Autodesk Inventor part; units mm, degrees
ref_plane "YZ Plane" through (0, 0, 0) normal (1, 0, 0) x (0, 1, 0)
ref_plane "XZ Plane" through (0, 0, 0) normal (0, 1, 0) x (-1, 0, 0)
ref_plane "XY Plane" through (0, 0, 0) normal (0, 0, 1) x (1, 0, 0)
sketch "Sketch1" plane through (0, 0, 0) normal (1, 0, 0) x (0, 1, 0)
  circle A0 centre (0, 0) radius 12.5
  circle A1 centre (-15.5, -15.5) radius 1.75
  circle A2 centre (15.5, -15.5) radius 1.75
  circle A3 centre (15.5, 15.5) radius 1.75
  circle A4 centre (-15.5, 15.5) radius 1.75
  line L0 (21.5, -21.5) -> (-21.5, -21.5)
  line L1 (-21.5, -21.5) -> (-21.5, 21.5)
  line L2 (-21.5, 21.5) -> (21.5, 21.5)
  line L3 (21.5, 21.5) -> (21.5, -21.5)
  line L4 (21.5, -21.5) -> (-21.5, 21.5) construction
  line L5 (-21.5, -21.5) -> (21.5, 21.5) construction
  dimension "d2" = 360
  dimension "d4" = 3.5
  dimension "d5" = 25
  dimension "d6" = 31
  dimension "d7" = 43
extrude "Extrusion1" add sketch "Sketch1" along normal blind 4
sketch "Sketch5" plane through (0, 21.5, 21.5) normal (0, 1, 0) x (1, 0, 0)
  line L0 (0, 43) -> (0, 0)
  line L1 (0, 0) -> (4, 0)
  line L2 (4, 43) -> (4, 0)
  line L3 (0, 43) -> (4, 43)
  line L4 (0, 43) -> (4, 43)
  line L5 (0, 43) -> (-18, 43)
  line L6 (-18, 43) -> (-18, 58)
  line L7 (-18, 58) -> (-15, 58)
  line L8 (-15, 58) -> (-15, 48)
  line L9 (-15, 48) -> (4, 48)
  line L10 (4, 48) -> (4, 43)
  line L11 (0, 0) -> (-18, 0)
  line L12 (-18, 0) -> (-18, -15)
  line L13 (-18, -15) -> (-15, -15)
  line L14 (-15, -15) -> (-15, -5)
  line L15 (-15, -5) -> (4, -5)
  line L16 (4, -5) -> (4, 0)
  line L17 (4, 43) -> (4, 0)
  point P0 (0, 21.5)
  dimension "d17" = 5
  dimension "d18" = 3
  dimension "d19" = 10
  dimension "d23" = 22
extrude "Extrusion4" add sketch "Sketch5" against normal up to surface (43 mm away) contours L5 L6 L7 L8 L9 L10 L3 | L1 L16 L15 L14 L13 L12 L11
sketch "Sketch6" plane through (-15, 21.5, 36.5) normal (1, 0, 0) x (0, 0, -1)
  line L0 (0, -43) -> (10, -43)
  line L1 (10, 0) -> (10, -43)
  line L2 (0, 0) -> (10, 0)
  line L3 (0, 0) -> (0, -43)
  line L4 (63, -43) -> (73, -43)
  line L5 (73, 0) -> (73, -43)
  line L6 (63, 0) -> (73, 0)
  line L7 (63, 0) -> (63, -43)
  point P0 (36.5, -21.5)
  point P1 (5, -6.5)
  point P2 (5, -36.5)
  point P3 (68, -36.5)
  point P4 (68, -6.5)
  point P5 (5, 0)
  point P6 (5, -43)
  point P7 (68, -43)
  point P8 (68, 0)
  dimension "d24" = 6.5
  dimension "d25" = 6.5
  dimension "d26" = 30
hole "Hole1" at (-15, 15, 31.5) at (-15, -15, 31.5) at (-15, -15, -31.5) at (-15, 15, -31.5) direction (-1, 0, 0) diameter 3.5 end through all
properties part number "Z Axis Motor Bracket" material "ABS Plastic"
CAD build for the part. Positions are in the model's coordinates, mm. A direction names the side the tool comes from. Give positions to 0.01 mm unless a question says otherwise; leave off trailing zeros. Write each loop counter-clockwise with the first axis right and the second up, starting at its lowest first coordinate (ties: lowest second). Pieces come first, ordered by that corner, then holes. Notation, with made-up numbers: (71, 44) -> (98, 44) arc R20 ccw to (98, 73) -> close; hole circle Ø6 at (-15, 69). An arc over 180 degrees is marked (long way). Write each question's results on one line, items separated by ' | '.
1. Cut at A-A, the plane y = 0. Write the cut outline in (x, z).
Geometry check:
outline: (-18, -36.5) -> (-15, -36.5) -> (-15, -26.5) -> (4, -26.5) -> (4, -12.5) -> (0, -12.5) -> (0, -21.5) -> (-18, -21.5) -> close; (-18, 21.5) -> (0, 21.5) -> (0, 12.5) -> (4, 12.5) -> (4, 26.5) -> (-15, 26.5) -> (-15, 36.5) -> (-18, 36.5) -> close
2. Drop flat-ended pins along their axis: P1, Ø9.5, axis at x = -2.5, y = 8.5, coming from the -Z side; P2, Ø8, axis at y = -4, z = 31, coming from the +X side; P3, Ø5.5, axis at y = -15.5, z = -15.5, coming from the -X side; P4, Ø3, axis at y = -15.5, z = 15.5, coming from the -X side. Give the stop position or say it passes through.
Geometry check:
P1: z = -26.5 | P2: x = -15 | P3: x = 0 | P4: through
3. Cut at C-C, the plane z = 0. Write the cut outline in (x, y), then the cut area to 3 significant figures.
Geometry check:
outline: (0, -21.5) -> (4, -21.5) -> (4, -12.5) -> (0, -12.5) -> close; (0, 12.5) -> (4, 12.5) -> (4, 21.5) -> (0, 21.5) -> close | area: 72.0 mm²
4. Cut at B-B, the plane x = -7.25. Write the cut outline in (y, z), then the cut area to 3 significant figures.
Geometry check:
outline: (-21.5, -26.5) -> (21.5, -26.5) -> (21.5, -21.5) -> (-21.5, -21.5) -> close; (-21.5, 21.5) -> (21.5, 21.5) -> (21.5, 26.5) -> (-21.5, 26.5) -> close | area: 430 mm²
5. Which spindle directions (+Z, -Z, +X, -X, +Y, -Y) get a long thin tool onto all of the face, cutting with end or side? Do faces 1 (the flat face through (0, 9, -9)), 2 (the flat face through (-6, 0, 26.5)), 3 (the flat face through (-15, 0, -32)). Say none if no direction does.
Geometry check:
face 1: -X, +Y, -Y | face 2: +Z, +X, +Y, -Y | face 3: -Z, +X, +Y, -Y
6. Cut at D-D, the plane z = -15.5. Write the cut outline in (x, y).
Geometry check:
outline: (0, -21.5) -> (4, -21.5) -> (4, -17.25) -> (0, -17.25) -> close; (0, -13.75) -> (4, -13.75) -> (4, 13.75) -> (0, 13.75) -> close; (0, 17.25) -> (4, 17.25) -> (4, 21.5) -> (0, 21.5) -> close
7. Wall check: probe 1 along Z at (x, y) = (2.8, -15.5); probe 2 along Y at (x, z) = (-17.15, -31.5); probe 3 along Z at (x, y) = (-15.6, 15). Give the ranges that are in metal, low to high. Write a range as [from, to].
Geometry check:
probe 1: [-26.5, -17.25], [-13.75, 13.75], [17.25, 26.5] | probe 2: [-21.5, -16.75], [-13.25, 13.25], [16.75, 21.5] | probe 3: [-36.5, -33.25], [-29.75, -21.5], [21.5, 29.75], [33.25, 36.5]
8. Two-plate mould, pull along Y, no slides. Class faces 4 (the cylindrical face through (-16.52, 13.82, -30.21)), 5 (the cylindrical face through (1.972, 15.272, 13.765)), 6 (the flat face through (0.2, -21.5, -0.5)), 7 (the flat face through (-18, 0, -29)): pulls with the +Y half, pulls with the -Y half, needs draft (parallel to the pull), parting line crosses it, or undercut.
Geometry check:
face 4: undercut | face 5: undercut | face 6: pulls with the -Y half | face 7: needs draft
